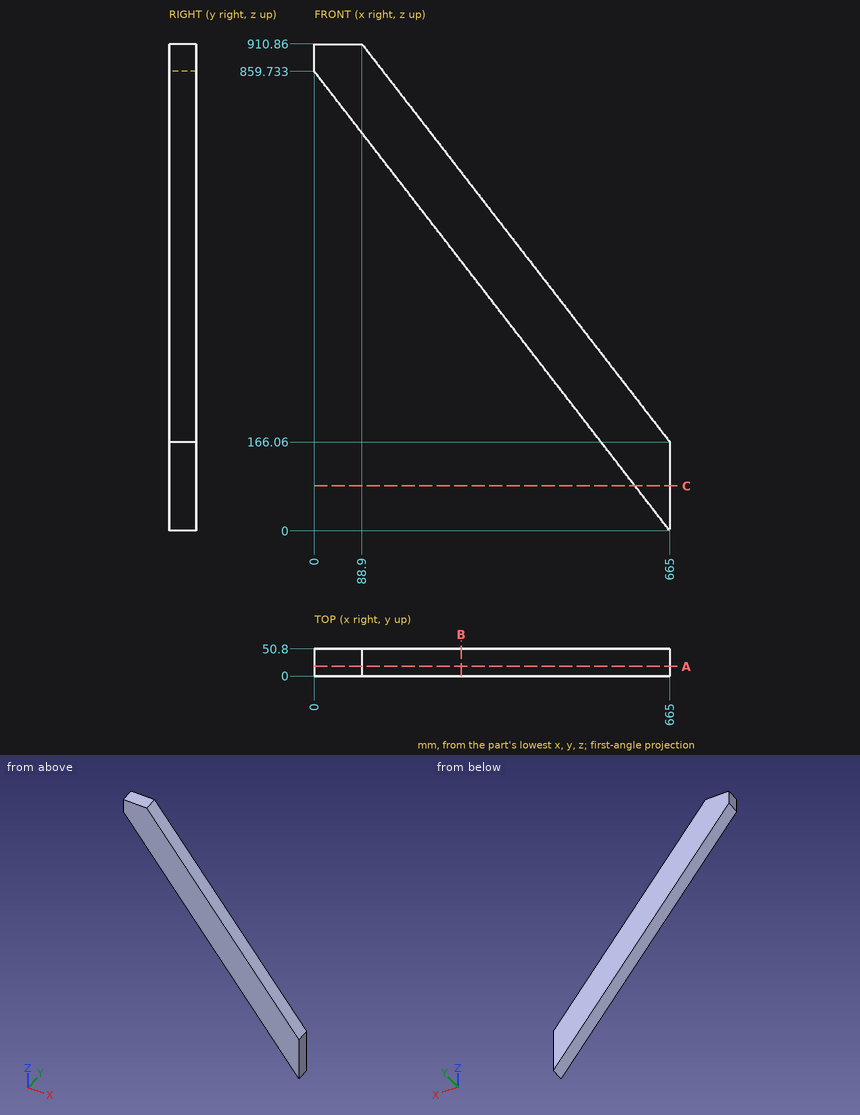
Print and shaded views of the part. All mm, measured from the part's lowest x, y and z. Round coordinates to 2 decimals unless told otherwise and drop trailing zeros. Write each loop counter-clockwise with the first axis right and the second up, starting at its lowest first coordinate (ties: lowest second). Pieces come first, ordered by that corner, then holes. Notation, with made-up numbers: M 12.25,-21 L 63.25,-21 A23 ccw 63.25,-6 Z; hole C 87,60 d11. An arc over 180 degrees is marked long. Use a Markdown table: item, result. Add a question column.
1. Slice it at C-C on z = 84. Give the cut face in (x, y), then the cut area to 3 significant figures.
2. Slice it at B-B on x = 274.5. Give the cut face in (y, z), then the cut area to 3 significant figures.
3. Drill centre lines: probe 1 along X at (y, z) = (14.5, 394.5) (1 decimal); probe 2 along X at (y, z) = (16.5, 771) (1 decimal); probe 3 along Z at (x, y) = (68.5, 7.5) (1 decimal). Where is each one in solid material? Low to high.
4. Slice it at A-A on y = 18. Give the cut face in (x, z), then the cut area to 3 significant figures.
5. Flat gauge pins, fed straight in: P1, Ø1, axis at x = 570.5, y = 16, coming from the -Z side (1 decimal); P2, Ø1.5, axis at x = 311.5, y = 20, coming from the -Z side (1 decimal); P3, Ø8, axis at y = 10.5, z = 706, coming from the -X side. Where does each tip first touch, or does it go through?
Reply:
| question | item | result |
|---|---|---|
| 1 | outline | M 600.03,0 L 665,0 L 665,50.8 L 600.03,50.8 Z |
| 1 | area | 3,300 mm^2 |
| 2 | outline | M 0,504.85 L 50.8,504.85 L 50.8,670.91 L 0,670.91 Z |
| 2 | area | 8,440 mm^2 |
| 3 | probe 1 | x = 359.9 to 488.3 |
| 3 | probe 2 | x = 68.6 to 197.1 |
| 3 | probe 3 | z = 771.2 to 910.9 |
| 4 | outline | M 0,859.73 L 665,0 L 665,166.06 L 88.9,910.86 L 0,910.86 Z |
| 4 | area | 105,000 mm^2 |
| 5 | P1 | stops at z = 121.5 |
| 5 | P2 | stops at z = 456 |
| 5 | P3 | stops at x = 115.82 |
